Can you work these out from the drawing? Everything is in mm from the part's minimum corner. A direction names the side the tool comes from. Coordinates: 2 decimals unless noted, no trailing zeros. Write each loop counter-clockwise with the first axis right and the second up, starting at its lowest first coordinate (ties: lowest second). Pieces come first, ordered by that corner, then holes. Notation, with made-up numbers: M 58,6.5 L 70,6.5 A34 cw 70,45.5 Z; hole C 82,17 d10. An arc over 180 degrees is marked long. Write item = value, one per line.
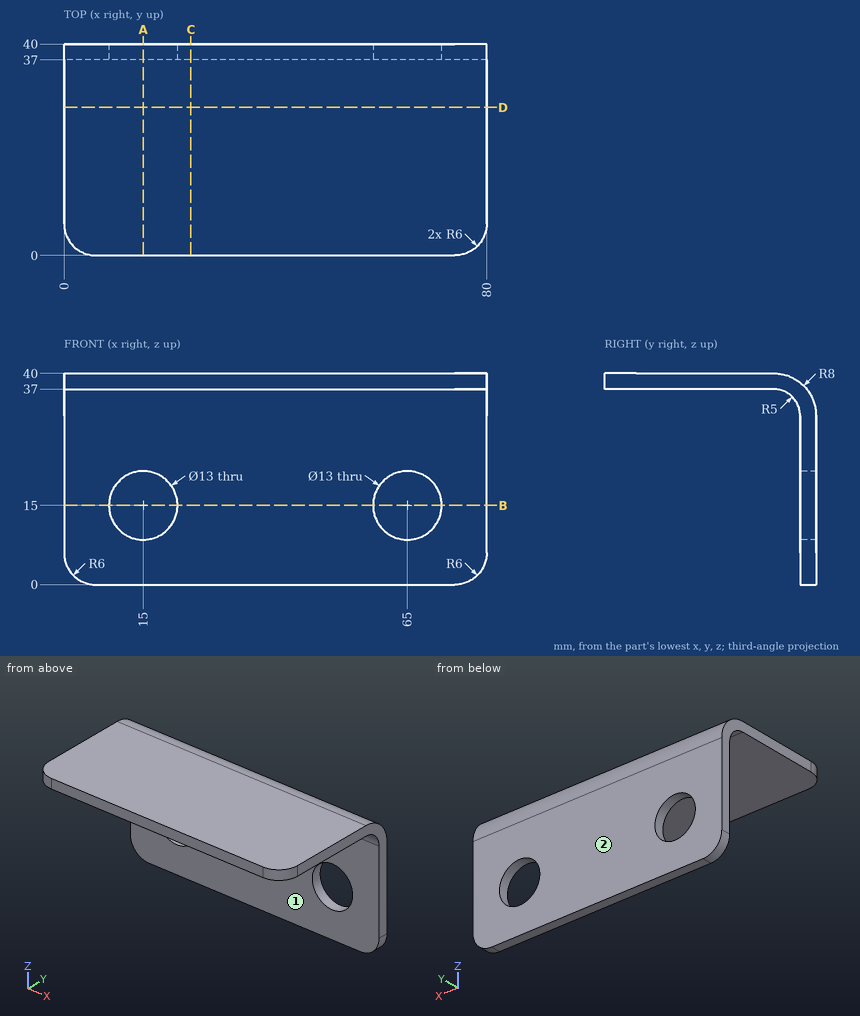
Item 1: Imagine slicing it at D-D (y = 28). Write out the boundary of the cut face in (x, z).
Numbers:
outline = M 0,37 L 80,37 L 80,40 L 0,40 Z
Item 2: Imagine slicing it at B-B (z = 15). Write out the boundary of the cut face in (x, y).
Numbers:
outline = M 0,37 L 8.5,37 L 8.5,40 L 0,40 Z; M 21.5,37 L 58.5,37 L 58.5,40 L 21.5,40 Z; M 71.5,37 L 80,37 L 80,40 L 71.5,40 Z
Item 3: Imagine slicing it at A-A (x = 15). Write out the boundary of the cut face in (y, z).
Numbers:
outline = M 0,37 L 32,37 A5 cw 37,32 L 37,21.5 L 40,21.5 L 40,32 A8 ccw 32,40 L 0,40 Z; M 37,0 L 40,0 L 40,8.5 L 37,8.5 Z
Item 4: For the marked faces 1 and 2, which set-ups out of +Z, -Z, +X, -X, +Y, -Y let a thin tool reach every point of the face, with its end or its side?
Numbers:
face_1 = -Z, +X, -X, -Y
face_2 = +Z, -Z, +X, -X, +Y
Item 5: If I drill on line 1 along Z through (x, y) = (7, 8); line 2 along Z through (x, y) = (15, 38), over which ranges is the centre line in solid material (lowest first)?
Numbers:
line_1 = 37 to 40
line_2 = 0 to 8.5, 21.5 to 37.29
Item 6: Imagine slicing it at C-C (x = 24). Write out the boundary of the cut face in (y, z), and give its area (3 significant figures).
Numbers:
outline = M 0,37 L 32,37 A5 cw 37,32 L 37,0 L 40,0 L 40,32 A8 ccw 32,40 L 0,40 Z
area = 223 mm²
Item 7: I'm going to push flat-ended pins straight in: P1, Ø1.5, axis at x = 33.5, y = 24, coming from the -Z side; P2, Ø9.5, axis at x = 58.5, z = 22, coming from the -Y side; P3, Ø1, axis at x = 12.5, z = 35, coming from the +Y side; P4, Ø11.5, axis at x = 65, z = 15, coming from the -Y side (1 decimal). Where does each tip first touch, or does it pass through?
Numbers:
P1 = 37
P2 = 37
P3 = 39.6
P4 = through
